```python
from build123d import *

# Parameters (mm, degrees)
BOSS_EXTRUDE1_DEPTH                     = 598
CBORE_FOR_M5_HEX_HEAD_BOLT1_D           = 3.5
CBORE_FOR_M5_HEX_HEAD_BOLT1_CBORE_D     = 6
CBORE_FOR_M5_HEX_HEAD_BOLT1_CBORE_DEPTH = 4.5
LPATTERN1_COUNT                         = 24
LPATTERN1_PITCH                         = 25.1


with BuildPart() as part:
    # Sketch1 → Boss-Extrude1 (new body)
    with BuildSketch(Plane.XY):
        with BuildLine():
            Line((0, 4), (-5.5, 4))
            Line((-5.5, 4), (-6, 3.5))
            Line((-6, 3.5), (-6, 3))
            ThreePointArc((-6, 3), (-5, 2), (-6, 1))
            Line((-6, 1), (-6, -3.5))
            Line((-6, -3.5), (-5.5, -4))
            Line((-5.5, -4), (5.5, -4))
            Line((5.5, -4), (6, -3.5))
            Line((6, -3.5), (6, 1))
            ThreePointArc((6, 1), (5, 2), (6, 3))
            Line((6, 3), (6, 3.5))
            Line((6, 3.5), (5.5, 4))
            Line((5.5, 4), (0, 4))
        make_face()
    extrude(amount=BOSS_EXTRUDE1_DEPTH)

    # CBORE for M5 Hex Head Bolt1 (through all)
    with Locations(Plane(origin=(0, 4, 0), x_dir=(1, 0, 0), z_dir=(0, 1, 0))):
        with Locations((0, -11)):
            cbore_for_m5_hex_head_bolt1 = CounterBoreHole(CBORE_FOR_M5_HEX_HEAD_BOLT1_D / 2, CBORE_FOR_M5_HEX_HEAD_BOLT1_CBORE_D / 2, CBORE_FOR_M5_HEX_HEAD_BOLT1_CBORE_DEPTH)

    # LPattern1: CBORE for M5 Hex Head Bolt1 ×24
    with Locations(*[(0, 0, i * LPATTERN1_PITCH) for i in range(1, LPATTERN1_COUNT)]):
        add(cbore_for_m5_hex_head_bolt1, mode=Mode.SUBTRACT)


solid = part.part
```
Can you work these out from the model? Positions are in its coordinate system, mm. Give positions to 0.01 mm unless a question says otherwise; leave off trailing zeros. Write each loop counter-clockwise with the first axis right and the second up, starting at its lowest first coordinate (ties: lowest second). Pieces come first, ordered by that corner, then holes. Notation, with made-up numbers: (70, 43.5) -> (118, 43.5) arc R30 ccw to (118, 67.5) -> close; hole circle Ø7 at (-8.75, 38.5). An arc over 180 degrees is marked (long way). One line per item, written item: value.
Q1. Imagine slicing it at B-B on z = 426.5. Please give me the cut outline in (x, y).
Results found:
outline: (-6, -3.5) -> (-5.5, -4) -> (5.5, -4) -> (6, -3.5) -> (6, 1) arc R1 cw to (6, 3) -> (6, 3.5) -> (5.5, 4) -> (-5.5, 4) -> (-6, 3.5) -> (-6, 3) arc R1 cw to (-6, 1) -> close
Q2. Please list where these lines run through material, in increasing order: line 1 (X direction, y = -2.5, z = 538); line 2 (X direction, y = 1.65, z = 563.2); line 3 (Y direction, x = -5.5, z = 316.5). Write a range as [from, to].
Results found:
line 1: x = [-6, -1.75], [1.75, 6]
line 2: x = [-5.06, -3], [3, 5.06]
line 3: y = [-4, 1.13], [2.87, 4]
Q3. Imagine slicing it at A-A on y = -2.25. Give the number of separate pieces and of enclosed holes in the cut face, and give its area (3 significant figures).
Results found:
separate pieces: 1
enclosed holes: 24
area: 6,950 mm^2
Q4. For P1, Ø3, axis at x = 0, z = 462.8, coming from the +Y side; P2, Ø3, axis at x = 0.5, z = 513.5, coming from the +Y side, each with a flat end and sliding along its axis, tell me the tip position at first contact or that it passes through.
Results found:
P1: passes through
P2: stops at y = -0.5
